```python
from build123d import *

# Parameters (mm, degrees)
SKETCH1_R           = 50
BOSS_EXTRUDE1_DEPTH = 2
SKETCH2_R           = 42.5
SKETCH2_R_2         = 36.25
CUT_EXTRUDE1_DEPTH  = 1
SKETCH3_R           = 1.5
CUT_EXTRUDE2_DEPTH  = 71.738956735
CHAMFER1_SIZE       = 2
CHAMFER1_SIZE2      = 1.154700538


with BuildPart() as part:
    # Sketch1 → Boss-Extrude1 (new body)
    with BuildSketch(Plane.XY):
        Circle(SKETCH1_R)
    extrude(amount=BOSS_EXTRUDE1_DEPTH)

    # Sketch2 → Cut-Extrude1 (cut)
    with BuildSketch(Plane.XY):
        Circle(SKETCH2_R)
        Circle(SKETCH2_R_2, mode=Mode.SUBTRACT)
    extrude(amount=CUT_EXTRUDE1_DEPTH, mode=Mode.SUBTRACT)

    # Sketch3 → Cut-Extrude2 (cut, through all)
    with BuildSketch(Plane(origin=(0, 0, 0), x_dir=(-1, 0, 0), z_dir=(0, 0, -1))):
        with Locations((0, 22.75)):
            Circle(SKETCH3_R)
        with Locations(Location((0, -22.75, 0), (0, 0, 180))):
            Circle(SKETCH3_R)
        with BuildLine():
            Line((-5, 27.041634566), (-5, 5))
            Line((-5, 5), (-27.041634566, 5))
            ThreePointArc((-27.041634566, 5), (-19.445436483, 19.445436483), (-5, 27.041634566))
        make_face()
        with BuildLine():
            Line((5, 27.041634566), (5, 5))
            Line((5, 5), (27.041634566, 5))
            ThreePointArc((27.041634566, 5), (19.445436483, 19.445436483), (5, 27.041634566))
        make_face()
        with BuildLine():
            Line((27.041634566, -5), (5, -5))
            Line((5, -5), (5, -27.041634566))
            ThreePointArc((5, -27.041634566), (19.445436483, -19.445436483), (27.041634566, -5))
        make_face()
        with BuildLine():
            Line((-5, -27.041634566), (-5, -5))
            Line((-5, -5), (-27.041634566, -5))
            ThreePointArc((-27.041634566, -5), (-19.445436483, -19.445436483), (-5, -27.041634566))
        make_face()
    extrude(amount=-CUT_EXTRUDE2_DEPTH, mode=Mode.SUBTRACT)

    # Chamfer1
    chamfer1_edges = [part.edges().sort_by_distance(p)[0] for p in [
        (1.5, 22.75, 0),
        (-1.5, -22.75, 0),
    ]]
    chamfer1_side = [part.faces().sort_by_distance(p)[0] for p in [
        (0, 0, 0),
    ]]
    chamfer(chamfer1_edges, length=CHAMFER1_SIZE, length2=CHAMFER1_SIZE2, reference=chamfer1_side[0])


solid = part.part
```
Could you check a few things on this model? Use its own coordinates, in mm. A direction names the side the tool comes from. Coordinates: 2 decimals unless noted, no trailing zeros. Write each loop counter-clockwise with the first axis right and the second up, starting at its lowest first coordinate (ties: lowest second). Pieces come first, ordered by that corner, then holes. Notation, with made-up numbers: (1, -11) -> (52, -11) arc R20 cw to (52, 21) -> close; hole circle Ø10 at (19.5, 50.25). An arc over 180 degrees is marked (long way). Return JSON: item names as keys, results as strings.
(1) I need wall thicknesses on L1, parallel to Y at x = 0, z = 1.75; L2, parallel to Y at x = 0, z = 0.3; L3, parallel to Y at x = 0, z = 0.35. Which ranges of each line are inside material? Lowest first, please.
Numbers:
{"L1": "y = -50 to -24.25, -21.25 to 21.25, 24.25 to 50", "L2": "y = -50 to -42.5, -36.25 to -25.73, -19.77 to 19.77, 25.73 to 36.25, 42.5 to 50", "L3": "y = -50 to -42.5, -36.25 to -25.64, -19.86 to 19.86, 25.64 to 36.25, 42.5 to 50"}
(2) Imagine slicing it at A-A, the plane x = 0. Please give me the cut outline in (y, z), then the cut area to 3 significant figures.
Numbers:
{"outline": "(-50, 0) -> (-42.5, 0) -> (-42.5, 1) -> (-36.25, 1) -> (-36.25, 0) -> (-26.25, 0) -> (-24.25, 1.15) -> (-24.25, 2) -> (-50, 2) -> close; (-21.25, 1.15) -> (-19.25, 0) -> (19.25, 0) -> (21.25, 1.15) -> (21.25, 2) -> (-21.25, 2) -> close; (24.25, 1.15) -> (26.25, 0) -> (36.25, 0) -> (36.25, 1) -> (42.5, 1) -> (42.5, 0) -> (50, 0) -> (50, 2) -> (24.25, 2) -> close", "area": "171 mm2"}
(3) Imagine slicing it at C-C, the plane y = 0. Please give me the cut outline in (x, z), then the cut area to 4 significant figures.
Numbers:
{"outline": "(-50, 0) -> (-42.5, 0) -> (-42.5, 1) -> (-36.25, 1) -> (-36.25, 0) -> (36.25, 0) -> (36.25, 1) -> (42.5, 1) -> (42.5, 0) -> (50, 0) -> (50, 2) -> (-50, 2) -> close", "area": "187.5 mm2"}
(4) Imagine slicing it at D-D, the plane y = 22.75. Please give me the cut outline in (x, z), then the cut area to 3 significant figures.
Numbers:
{"outline": "(-44.52, 0) -> (-35.9, 0) -> (-35.9, 1) -> (-28.22, 1) -> (-28.22, 0) -> (-15.45, 0) -> (-15.45, 2) -> (-44.52, 2) -> close; (-5, 0) -> (-3.5, 0) -> (-1.5, 1.15) -> (-1.5, 2) -> (-5, 2) -> close; (1.5, 1.15) -> (3.5, 0) -> (5, 0) -> (5, 2) -> (1.5, 2) -> close; (15.45, 0) -> (28.22, 0) -> (28.22, 1) -> (35.9, 1) -> (35.9, 0) -> (44.52, 0) -> (44.52, 2) -> (15.45, 2) -> close", "area": "113 mm2"}
(5) Imagine slicing it at B-B, the plane z = 1.5. Please give me the cut outline in (x, y), then the cut area to 3 significant figures.
Numbers:
{"outline": "circle Ø100 at (0, 0); hole (-27.04, -5) arc R27.5 ccw to (-5, -27.04) -> (-5, -5) -> close; hole (-27.04, 5) -> (-5, 5) -> (-5, 27.04) arc R27.5 ccw to start; hole circle Ø3 at (0, -22.75); hole circle Ø3 at (0, 22.75); hole (5, -27.04) arc R27.5 ccw to (27.04, -5) -> (5, -5) -> close; hole (5, 5) -> (27.04, 5) arc R27.5 ccw to (5, 27.04) -> close", "area": "6,460 mm2"}
(6) We'd pull the mould along Y, two halves only. Please class faces 1 (the cylindrical face through (47.69, 15.02, 0.99)), 2 (the cylindrical face through (-0.195, -24.237, 1.571)), 3 (the flat face through (-1, 1, 2)): +Y half, -Y half, draft (parallel to the pull), parting line (faces both ways), or undercut.
Numbers:
{"face 1": "parting line", "face 2": "undercut", "face 3": "draft"}
(7) Which directions (+Z, -Z, +X, -X, +Y, -Y) give clear straight access to the entire face, cutting with the end or side of a thin tool? Please do faces 4 (the cylindrical face through (-33.727, -25.861, 0.493)), 5 (the flat face through (-22, -37, 0)).
Numbers:
{"face 4": "-Z", "face 5": "-Z, +X, -X, +Y, -Y"}
(8) I'm going to push flat-ended pins straight in: pin 1 (0.6 mm diameter, centred on y = 20, z = 1, fed in from +X); pin 2 (0.6 mm diameter, centred on y = 14.5, z = 1, fed in from -X); pin 3 (3.5 mm diameter, centred on x = 0, y = 22.75, fed in from -Z). Where does each tip first touch, or does it pass through?
Numbers:
{"pin 1": "stops at x = 45.96", "pin 2": "stops at x = -47.94", "pin 3": "stops at z = 1.01"}
